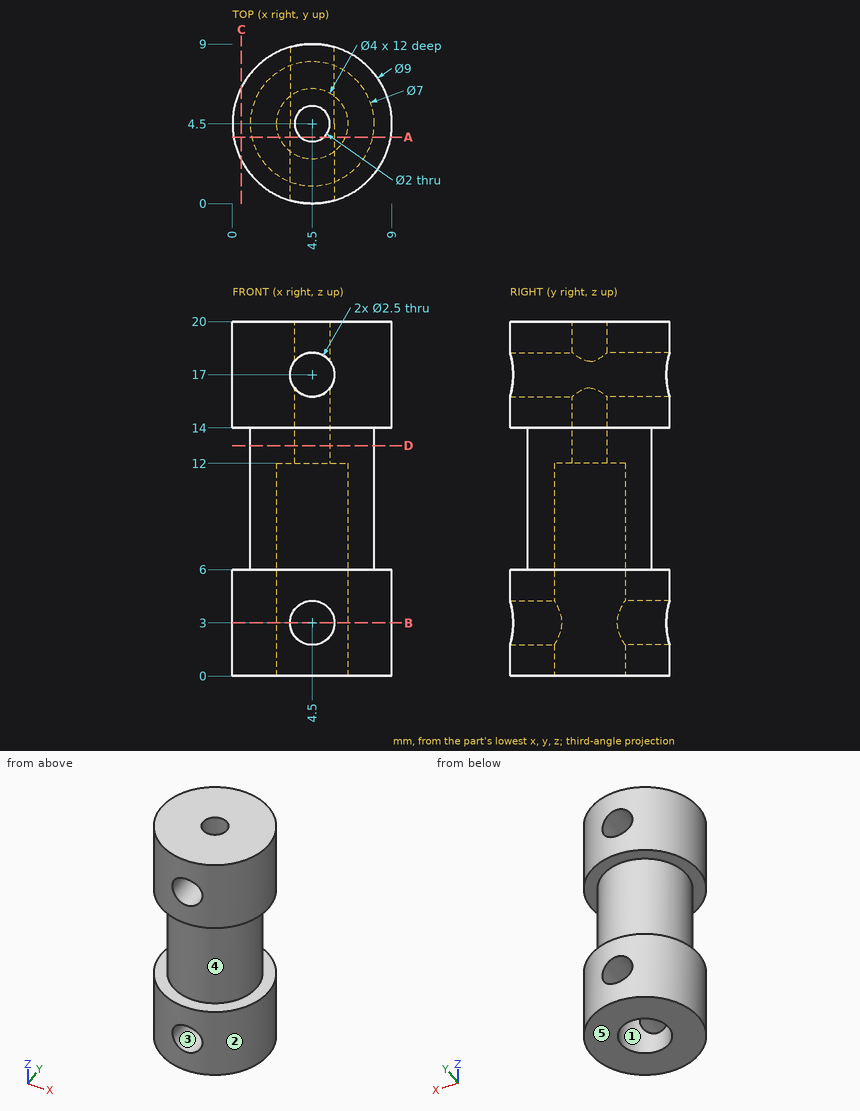
Can you work these out from the drawing? Everything is in mm from the part's minimum corner. A direction names the side the tool comes from. Coordinates: 2 decimals unless noted, no trailing zeros. Write each loop counter-clockwise with the first axis right and the second up, starting at its lowest first coordinate (ties: lowest second). Pieces come first, ordered by that corner, then holes. Notation, with made-up numbers: (27, 87) -> (38, 87) arc R26 cw to (38, 110) -> close; hole circle Ø9 at (11, -19.5). An arc over 180 degrees is marked (long way). Write each question's results on one line, items separated by ' | '. Start each with the question number.
Q1. Imagine slicing it at C-C (x = 0.5). Write out the boundary of the cut face in (y, z), then the cut area to 3 significant figures.
Q2. If I drill on probe 1 along Z at (x, y) = (4.5, 2.35); probe 2 along Z at (x, y) = (7.25, 2); probe 3 along Z at (x, y) = (3.5, 5.25), over which ranges is the centre line in solid material (lowest first)?
Q3. I'm going to push flat-ended pins straight in: pin 1 (1 mm diameter, centred on x = 1.5, z = 3, fed in from +Y); pin 2 (1.5 mm diameter, centred on x = 4, z = 7, fed in from +Y). Where does each tip first touch, or does it pass through?
Q4. Imagine slicing it at A-A (y = 3.75). Write out the boundary of the cut face in (x, z).
Q5. We'd pull the mould along X, two halves only. Please class the marked faces 3, 4 and 5: +X half, -X half, draft (parallel to the pull), parting line (faces both ways), or undercut.
Q6. On a 3-axis mill with a long thin cutter (end or side, diameter ignored), from which of +Z, -Z, +X, -X, +Y, -Y can I reach the whole of each face in a straight line? I mean the marked faces 1 and 2. Say none if no direction works.
Q7. Imagine slicing it at B-B (z = 3). Write out the boundary of the cut face in (x, y).
Q8. Imagine slicing it at D-D (z = 13). Write out the boundary of the cut face in (x, y), then the cut area to 3 significant figures.
Taken from the geometry:
1) outline: (2.44, 0) -> (6.56, 0) -> (6.56, 6) -> (2.44, 6) -> close; (2.44, 14) -> (6.56, 14) -> (6.56, 20) -> (2.44, 20) -> close | area: 49.5 mm^2
2) probe 1: z = 0 to 1.75, 4.25 to 15.75, 18.25 to 20 | probe 2: z = 0 to 6, 14 to 20 | probe 3: z = 12 to 16.25, 17.75 to 20
3) pin 1: stops at y = 8.24 | pin 2: stops at y = 8
4) outline: (0.06, 0) -> (2.65, 0) -> (2.65, 12) -> (3.84, 12) -> (3.84, 15.94) arc R1.25 cw to (3.84, 18.06) -> (3.84, 20) -> (0.06, 20) -> (0.06, 14) -> (1.08, 14) -> (1.08, 6) -> (0.06, 6) -> close; (5.16, 12) -> (6.35, 12) -> (6.35, 0) -> (8.94, 0) -> (8.94, 6) -> (7.92, 6) -> (7.92, 14) -> (8.94, 14) -> (8.94, 20) -> (5.16, 20) -> (5.16, 18.06) arc R1.25 cw to (5.16, 15.94) -> close
5) face 3: undercut | face 4: parting line | face 5: draft
6) face 1: -Z | face 2: +Z, -Z
7) outline: (3.25, 0.18) -> (3.25, 2.94) arc R2 cw to (3.25, 6.06) -> (3.25, 8.82) arc R4.5 ccw to start; (5.75, 0.18) arc R4.5 ccw to (5.75, 8.82) -> (5.75, 6.06) arc R2 cw to (5.75, 2.94) -> close
8) outline: circle Ø7 at (4.5, 4.5); hole circle Ø2 at (4.5, 4.5) | area: 35.3 mm^2
